Part print with two shaded views. Sizes in mm from the minimum x, y, z corner. Give positions to 0.01 mm unless a question says otherwise; leave off trailing zeros. Loops run counter-clockwise (first coordinate to the right, second up) from the corner with the lowest first, then second, coordinate; pieces in that order, holes last. Notation, with made-up numbers: M -40,-16 L -14,-16 A20 ccw -14,20 Z; hole C 85.25,-20.75 d4. An arc over 180 degrees is marked long. Answer as a JSON object with one key per item and string values. Group by question number.
1. Slice it at D-D (z = 25). List the corners of the cut face in (x, y).
2. Slice it at C-C (z = 7.45). List the corners of the cut face in (x, y), then the cut area to 3 significant figures.
3. Slice it at B-B (x = 2.15). List the corners of the cut face in (y, z), then the cut area to 3 significant figures.
4. Drill centre lines: line 1 along Z through (x, y) = (0.3, 18); line 2 along Y through (x, z) = (2.3, 7.45); line 3 along Z through (x, y) = (1.05, 32). Where is each one in solid material? Low to high. Write a range as [from, to].
5. Slice it at A-A (y = 35.95). List the corners of the cut face in (x, z), then the cut area to 3 significant figures.
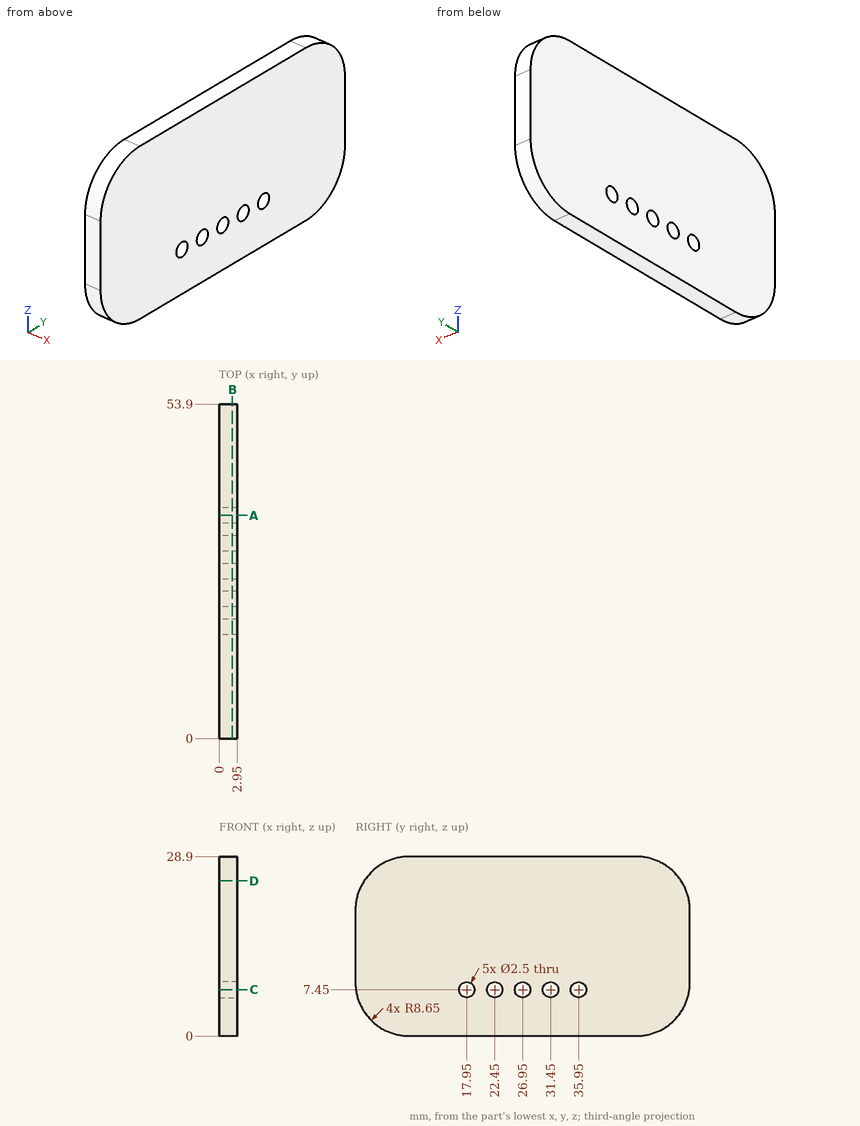
Established:
{
 "1": {"outline": "M 0,1.42 L 2.95,1.42 L 2.95,52.48 L 0,52.48 Z"},
 "2": {"outline": "M 0,0.08 L 2.95,0.08 L 2.95,16.7 L 0,16.7 Z; M 0,19.2 L 2.95,19.2 L 2.95,21.2 L 0,21.2 Z; M 0,23.7 L 2.95,23.7 L 2.95,25.7 L 0,25.7 Z; M 0,28.2 L 2.95,28.2 L 2.95,30.2 L 0,30.2 Z; M 0,32.7 L 2.95,32.7 L 2.95,34.7 L 0,34.7 Z; M 0,37.2 L 2.95,37.2 L 2.95,53.82 L 0,53.82 Z", "area": "122 mm^2"},
 "3": {"outline": "M 0,8.65 A8.65 ccw 8.65,0 L 45.25,0 A8.65 ccw 53.9,8.65 L 53.9,20.25 A8.65 ccw 45.25,28.9 L 8.65,28.9 A8.65 ccw 0,20.25 Z; hole C 17.95,7.45 d2.5; hole C 22.45,7.45 d2.5; hole C 26.95,7.45 d2.5; hole C 31.45,7.45 d2.5; hole C 35.95,7.45 d2.5", "area": "1,470 mm^2"},
 "4": {"line 1": "z = [0, 6.2], [8.7, 28.9]", "line 2": "y = [0.08, 16.7], [19.2, 21.2], [23.7, 25.7], [28.2, 30.2], [32.7, 34.7], [37.2, 53.82]", "line 3": "z = [0, 6.33], [8.57, 28.9]"},
 "5": {"outline": "M 0,0 L 2.95,0 L 2.95,6.2 L 0,6.2 Z; M 0,8.7 L 2.95,8.7 L 2.95,28.9 L 0,28.9 Z", "area": "77.9 mm^2"}
}
